from build123d import *

# Parameters (mm, degrees)
SKETCH1_R             = 5
CORPO_DEPTH           = 10
SKETCH2_R             = 1.5
FURO_3_PASSANTE_DEPTH = 45.158804332


with BuildPart() as part:
    # Sketch1 → Corpo (new body)
    with BuildSketch(Plane.XY):
        with BuildLine():
            Line((-12.5, -33.412291828), (-12.5, 33.412291828))
            ThreePointArc((-12.5, 33.412291828), (0, 35), (12.5, 33.412291828))
            Line((12.5, 33.412291828), (12.5, -33.412291828))
            ThreePointArc((12.5, -33.412291828), (0, -35), (-12.5, -33.412291828))
        make_face()
        with Locations((0, -25)):
            Circle(SKETCH1_R, mode=Mode.SUBTRACT)
        with Locations((0, 25)):
            Circle(SKETCH1_R, mode=Mode.SUBTRACT)
    extrude(amount=CORPO_DEPTH)

    # Sketch2 → Furo Ø3 Passante (cut, through all)
    with BuildSketch(Plane(origin=(12.5, 0, 0), x_dir=(0, 0, -1), z_dir=(1, 0, 0))):
        with Locations(Location((-5, 25, 0), (0, 0, 90))):
            Circle(SKETCH2_R)
    extrude(amount=-FURO_3_PASSANTE_DEPTH, mode=Mode.SUBTRACT)


solid = part.part
The model under review builds one solid part; all positions refer to its coordinate system, in mm. Give positions to 0.01 mm unless a question says otherwise; leave off trailing zeros. Order: outer loops, then holes, each group sorted by start corner. A loop starts at its lowest first (then second) coordinate and runs counter-clockwise, first axis right, second up. Notation, with made-up numbers: (-26.5, -5.5) -> (-19.5, -5.5) arc R19 ccw to (-19.5, 12.5) -> close; hole circle Ø9 at (-17, -15.5). An arc over 180 degrees is marked (long way). Write item = value, one per line. Start each with the question number.
(1) Take a section at B-B (z = 5). Write out the cut boundary in (x, y), plus the area to 3 significant figures.
(2) Take a section at A-A (y = -25). Write out the cut boundary in (x, z).
(3) For pin 1 Ø1.8 at (y, z) = (25, 5) entering from +X; pin 2 Ø3 at (x, z) = (-3, 8.5) entering from -Y, all flat-tipped, find the tip position at first contact; note any pin that passes through.
(4) Take a section at C-C (x = 0). Write out the cut boundary in (y, z), plus the area to 3 significant figures.
(5) Draft analysis for pull direction X (two halves, no side actions). For faces 1 (the cylindrical face through (0, -35, 5)), 2 (the cylindrical face through (-8.58, 23.5, 5.07)), 3 (the flat face through (12.5, 0, 5)), 4 (the cylindrical face through (4.619, 23.085, 4.93)), state which applies: +X half, -X half, draft (parallel to the pull), parting line (faces both ways), or undercut.
(6) Take a section at D-D (y = 25). Write out the cut boundary in (x, z).
(7) For L1, parallel to Y at x = 0, z = 7.25; L2, parallel to Z at x = 8.5, y = 25; L3, parallel to Y at x = 0.75, z = 9, list the stretches that pass through material, from the lowest coordinate up. Write a range as from..to.
Returned:
q1.outline = (-12.5, -33.41) arc R50 ccw to (12.5, -33.41) -> (12.5, 23.5) -> (4.77, 23.5) arc R5 cw to (-4.77, 23.5) -> (-12.5, 23.5) -> close; (-12.5, 26.5) -> (-4.77, 26.5) arc R5 cw to (4.77, 26.5) -> (12.5, 26.5) -> (12.5, 33.41) arc R50 ccw to (-12.5, 33.41) -> close; hole circle Ø10 at (0, -25)
q1.area = 1,520 mm²
q2.outline = (-12.5, 0) -> (-5, 0) -> (-5, 10) -> (-12.5, 10) -> close; (5, 0) -> (12.5, 0) -> (12.5, 10) -> (5, 10) -> close
q3.pin_1 = through
q3.pin_2 = -34.98
q4.outline = (-35, 0) -> (-30, 0) -> (-30, 10) -> (-35, 10) -> close; (-20, 0) -> (20, 0) -> (20, 10) -> (-20, 10) -> close; (30, 0) -> (35, 0) -> (35, 10) -> (30, 10) -> close
q4.area = 500 mm²
q5.face_1 = parting line
q5.face_2 = draft
q5.face_3 = +X half
q5.face_4 = undercut
q6.outline = (-12.5, 0) -> (-5, 0) -> (-5, 3.5) -> (-12.5, 3.5) -> close; (-12.5, 6.5) -> (-5, 6.5) -> (-5, 10) -> (-12.5, 10) -> close; (5, 0) -> (12.5, 0) -> (12.5, 3.5) -> (5, 3.5) -> close; (5, 6.5) -> (12.5, 6.5) -> (12.5, 10) -> (5, 10) -> close
q7.L1 = -35..-30, -20..20, 30..35
q7.L2 = 0..3.5, 6.5..10
q7.L3 = -34.99..-29.94, -20.06..20.06, 29.94..34.99
